Geometry: final body of the model. Coordinates: model frame, mm. Face numbers are marked on the shaded views. A direction names the side the tool comes from. Coordinates: 2 decimals unless noted, no trailing zeros. Order: outer loops, then holes, each group sorted by start corner. A loop starts at its lowest first (then second) coordinate and runs counter-clockwise, first axis right, second up. Notation, with made-up numbers: (1, 84.25) -> (8, 84.25) arc R22 cw to (8, 121.25) -> close; hole circle Ø5 at (24.25, -5.5). An arc over 180 degrees is marked (long way). Answer in a Markdown table with one row per item. Add a question column.
1) Section query D-D on y = 4.75. Return the cut outline in (x, z).
2) Contact query for flat-ended pins moving along their axis: P1, Ø3, axis at x = -6.5, y = -3.5, coming from the +Z side; P2, Ø2, axis at x = 3, z = -1, coming from the -Y side; P3, Ø2, axis at y = -2.5, z = -2.5, coming from the +X side. Output: stop coordinate, or through.
3) Section query C-C on x = 7.5. Return the cut outline in (y, z), then the cut area to 3 significant figures.
4) Ray query, line 1 (X direction, y = 1.75, z = -3.65); line 2 (Z direction, x = -8, y = -4.25); line 3 (Y direction, x = -10, z = -2.6). Return the intervals inside material, ascending. Write a range as from..to.
5) Section query B-B on y = -2.75. Return the cut outline in (x, z), then the cut area to 3 significant figures.
6) Set-up query: the marked faces 5 and 6. Return all of +Z, -Z, +X, -X, +Y, -Y with unobstructed straight access to the full face (end or side cutting, diameter ignored); none if empty.
7) Pull-direction query (X, two-part tool) for the marked faces 1, 2, 3 and 4; classes: +X half, -X half, draft (parallel to the pull), parting line (faces both ways), or undercut.
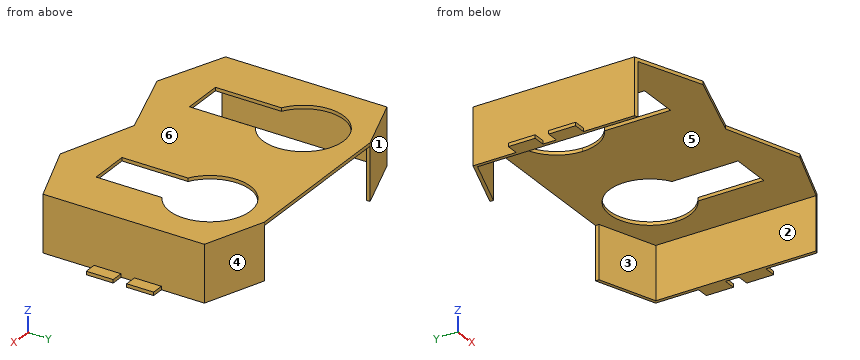
```python
from build123d import *

# Parameters (mm, degrees)
F1_DEPTH = 4.2
F3_DEPTH = 3.95
F4_W     = 0.9
F4_H     = 3.95
F5_DEPTH = 9.801


with BuildPart() as f1:
    # F0 (on Top) → F1 (new body)
    with BuildSketch(Plane.XY):
        Polygon((-6.102773, 6.8), (-10.55, 5.197539), (-10.55, 2), (-11.45, 2), (-11.45, 0), (-10.55, 0), (-10.55, -1), (-11.45, -1), (-11.45, -3), (-10.55, -3), (-10.55, -6.793472), (-5.599174, -8.7), (0, -6.793472), (0, 0), (0, 6.8), align=None)
        with BuildLine():
            ThreePointArc((-6.895583, -0.298076), (-6.895583, 4.898076), (-2.395583, 2.3))
            ThreePointArc((-2.395583, 2.3), (-2.797507, 0.8), (-3.895583, -0.298076))
            Line((-3.895583, -0.298076), (-3.895583, -5.2))
            Line((-3.895583, -5.2), (-5.395583, -5.2))
            Line((-5.395583, -5.2), (-6.895583, -5.2))
            Line((-6.895583, -5.2), (-6.895583, -0.298076))
        make_face(mode=Mode.SUBTRACT)
        Polygon((6.102773, 6.8), (0, 6.8), (0, 0), (0, -6.793472), (5.599174, -8.7), (10.55, -6.793472), (10.55, -3), (11.45, -3), (11.45, -1), (10.55, -1), (10.55, 0), (11.45, 0), (11.45, 2), (10.55, 2), (10.55, 5.197539), align=None)
        with BuildLine():
            ThreePointArc((3.895583, -0.298076), (3.895583, 4.898076), (8.395583, 2.3))
            ThreePointArc((8.395583, 2.3), (7.99366, 0.8), (6.895583, -0.298076))
            Line((6.895583, -0.298076), (6.895583, -5.2))
            Line((6.895583, -5.2), (5.395583, -5.2))
            Line((5.395583, -5.2), (3.895583, -5.2))
            Line((3.895583, -5.2), (3.895583, -0.298076))
        make_face(mode=Mode.SUBTRACT)
    extrude(amount=-F1_DEPTH)

    # F2 (on face) → F3 (cut)
    with BuildSketch(Plane(origin=(0, 0, -4.2), x_dir=(1, 0, 0), z_dir=(0, 0, -1))):
        Polygon((10.3, -5.021887), (10.3, 9.377568), (0, 9.377568), (-10.3, 9.37597), (-10.297766, -5.023484), (-6.100304, -6.535212), (-6.099994, -8.536118), (0.001405, -8.73276), (6.102773, -8.535172), (6.102773, -6.534266), align=None)
    extrude(amount=-F3_DEPTH, mode=Mode.SUBTRACT)

    # F4 (on face) → F5 (cut, through all)
    with BuildSketch(Plane.XZ.offset(3)):
        with Locations((-11, -1.975)):
            Rectangle(F4_W, F4_H)
        with Locations((11, -1.975)):
            Rectangle(F4_W, F4_H)
    extrude(amount=-F5_DEPTH, mode=Mode.SUBTRACT)


solid = f1.part
```
Result:
| question | item | result |
|---|---|---|
| 1 | outline | (-10.55, -4.2) -> (-10.3, -4.2) -> (-10.3, -0.25) -> (-7.13, -0.25) -> (-7.13, 0) -> (-10.55, 0) -> close; (-3.66, -0.25) -> (3.66, -0.25) -> (3.66, 0) -> (-3.66, 0) -> close; (7.13, -0.25) -> (10.3, -0.25) -> (10.3, -4.2) -> (10.55, -4.2) -> (10.55, 0) -> (7.13, 0) -> close |
| 2 | P1 | z = 0 |
| 2 | P2 | y = -8.04 |
| 2 | P3 | x = 10.55 |
| 3 | outline | (-7.97, -0.25) -> (0.16, -0.25) -> (0.16, 0) -> (-7.97, 0) -> close; (4.44, -0.25) -> (6.03, -0.25) -> (6.03, -4.2) -> (6.3, -4.2) -> (6.3, 0) -> (4.44, 0) -> close |
| 3 | area | 3.55 mm2 |
| 4 | line 1 | -10.55..-10.3, 10.3..10.55 |
| 4 | line 2 | -0.25..0 |
| 4 | line 3 | 5.13..5.4 |
| 5 | outline | (-11.45, -4.2) -> (-10.3, -4.2) -> (-10.3, -0.25) -> (-6.9, -0.25) -> (-6.9, 0) -> (-10.55, 0) -> (-10.55, -3.95) -> (-11.45, -3.95) -> close; (-3.9, -0.25) -> (3.9, -0.25) -> (3.9, 0) -> (-3.9, 0) -> close; (6.9, -0.25) -> (10.3, -0.25) -> (10.3, -4.2) -> (11.45, -4.2) -> (11.45, -3.95) -> (10.55, -3.95) -> (10.55, 0) -> (6.9, 0) -> close |
| 5 | area | 6.20 mm2 |
| 6 | face 5 | -Z, -Y |
| 6 | face 6 | +Z, +X, -X, +Y, -Y |
| 7 | face 1 | -X half |
| 7 | face 2 | undercut |
| 7 | face 3 | undercut |
| 7 | face 4 | +X half |
